Part model, mm, in its own coordinate system. Coordinates: 2 decimals unless noted, no trailing zeros. Loops run counter-clockwise (first coordinate to the right, second up) from the corner with the lowest first, then second, coordinate; pieces in that order, holes last. Notation, with made-up numbers: (-25.75, 15) - (31.25, 15) arc R26 ccw to (31.25, 49) - close; hole circle Ø6 at (-18.75, -30.75). An arc over 180 degrees is marked (long way). Answer as CSV lines item,"result".
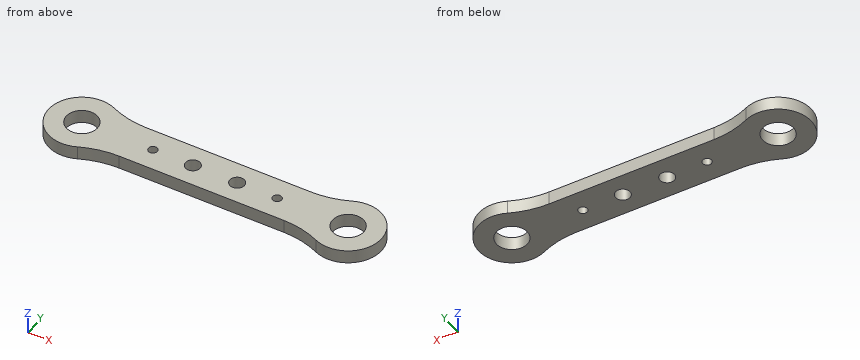
from build123d import *

# Parameters (mm, degrees)
ESBO_O1_R                = 1
ESBO_O1_R_2              = 3.5
ESBO_O1_R_3              = 1.65
RESSALTO_EXTRUS_O1_DEPTH = 3
FILETE1_R                = 20


with BuildPart() as part:
    # Esboço1 → Ressalto-extrusão1 (new body)
    with BuildSketch(Plane.XY):
        with BuildLine():
            Line((5.590169944, -5), (54.409830056, -5))
            ThreePointArc((54.409830056, -5), (67.5, 0), (54.409830056, 5))
            Line((54.409830056, 5), (5.590169944, 5))
            ThreePointArc((5.590169944, 5), (-7.5, 0), (5.590169944, -5))
        make_face()
        with Locations((44, 0)):
            Circle(ESBO_O1_R, mode=Mode.SUBTRACT)
        with Locations((16, 0)):
            Circle(ESBO_O1_R, mode=Mode.SUBTRACT)
        Circle(ESBO_O1_R_2, mode=Mode.SUBTRACT)
        with Locations((60, 0)):
            Circle(ESBO_O1_R_2, mode=Mode.SUBTRACT)
        with Locations((25, 0)):
            Circle(ESBO_O1_R_3, mode=Mode.SUBTRACT)
        with Locations((35, 0)):
            Circle(ESBO_O1_R_3, mode=Mode.SUBTRACT)
    extrude(amount=RESSALTO_EXTRUS_O1_DEPTH)

    # Filete1
    filete1_edges = [part.edges().sort_by_distance(p)[0] for p in [
        (54.409830056, -5, 1.5),
        (5.590169944, -5, 1.5),
        (5.590169944, 5, 1.5),
        (54.409830056, 5, 1.5),
    ]]
    fillet(filete1_edges, radius=FILETE1_R)


solid = part.part
Q1. Saw through at B-B (x = 16). Give the cut face in (y, z).
Results:
outline,"(-5, 0) - (-1, 0) - (-1, 3) - (-5, 3) - close; (1, 0) - (5, 0) - (5, 3) - (1, 3) - close"
Q2. Wall check: L1, parallel to Y at x = 44, z = 2.1; L2, parallel to X at y = 2.5, z = 0.8; L3, parallel to Y at x = 25, z = 1.35. Give the ranges that are in metal, low to high.
Results:
L1,"y = -5 to -1, 1 to 5"
L2,"x = -7.07 to -2.45, 2.45 to 57.55, 62.45 to 67.07"
L3,"y = -5 to -1.65, 1.65 to 5"
Q3. Saw through at A-A (y = 0). Give the cut face in (x, z).
Results:
outline,"(-7.5, 0) - (-3.5, 0) - (-3.5, 3) - (-7.5, 3) - close; (3.5, 0) - (15, 0) - (15, 3) - (3.5, 3) - close; (17, 0) - (23.35, 0) - (23.35, 3) - (17, 3) - close; (26.65, 0) - (33.35, 0) - (33.35, 3) - (26.65, 3) - close; (36.65, 0) - (43, 0) - (43, 3) - (36.65, 3) - close; (45, 0) - (56.5, 0) - (56.5, 3) - (45, 3) - close; (63.5, 0) - (67.5, 0) - (67.5, 3) - (63.5, 3) - close"
Q4. Saw through at C-C (z = 0.6). Give the cut face in (x, y).
Results:
outline,"(3.12, -6.82) arc R20 cw to (11.46, -5) - (48.54, -5) arc R20 cw to (56.88, -6.82) arc R7.5 ccw (long way) to (56.88, 6.82) arc R20 cw to (48.54, 5) - (11.46, 5) arc R20 cw to (3.12, 6.82) arc R7.5 ccw (long way) to start; hole circle Ø7 at (0, 0); hole circle Ø2 at (16, 0); hole circle Ø3.3 at (25, 0); hole circle Ø3.3 at (35, 0); hole circle Ø2 at (44, 0); hole circle Ø7 at (60, 0)"
Q5. Flat gauge pins, fed straight in: pin 1 (1.5 mm diameter, centred on x = 30, z = 1, fed in from -Y); pin 2 (1.5 mm diameter, centred on x = 25, z = 2, fed in from +Y). Where does each tip first touch, or does it go through?
Results:
pin 1,"stops at y = -5"
pin 2,"stops at y = 5"
Q6. Saw through at D-D (x = -0.5). Give the cut face in (y, z).
Results:
outline,"(-7.48, 0) - (-3.46, 0) - (-3.46, 3) - (-7.48, 3) - close; (3.46, 0) - (7.48, 0) - (7.48, 3) - (3.46, 3) - close"
